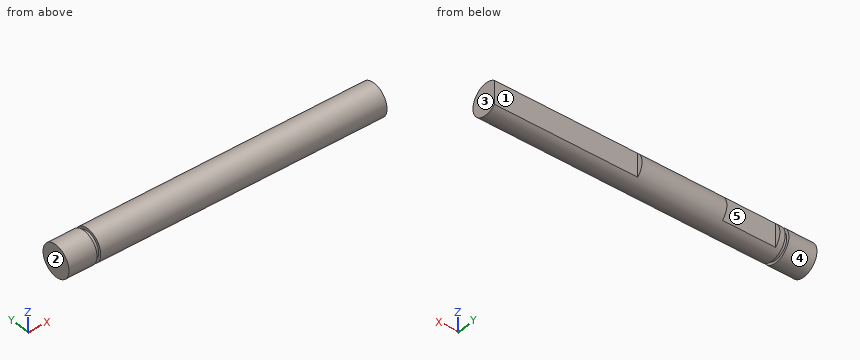
```python
from build123d import *

# Parameters (mm, degrees)
ESQUISSE2_W             = 10
ESQUISSE2_H             = 6
ESQUISSE2_W_2           = 27
ENL_V_MAT_EXTRU_1_DEPTH = 1


with BuildPart() as part:
    # Esquisse1 → Révolution1 (revolve)
    with BuildSketch(Plane.XY):
        Polygon((0, 0), (0, 3), (5.3, 3), (5.3, 2.5), (6, 2.5), (6, 3), (60, 3), (60, 0), align=None)
    revolve(axis=Axis((60, 0, 0), (-1, 0, 0)))

    # Esquisse2 → Enlèv. mat.-Extru.1 (cut)
    with BuildSketch(Plane(origin=(0, 3, 0), x_dir=(1, 0, 0), z_dir=(0, 1, 0))):
        with Locations((12, 0)):
            Rectangle(ESQUISSE2_W, ESQUISSE2_H)
        with Locations((46.5, 0)):
            Rectangle(ESQUISSE2_W_2, ESQUISSE2_H)
    extrude(amount=-ENL_V_MAT_EXTRU_1_DEPTH, mode=Mode.SUBTRACT)


solid = part.part
```
Could you check a few things on this model? Use its own coordinates, in mm. Face numbers are marked on the shaded views. A direction names the side the tool comes from. Coordinates: 2 decimals unless noted, no trailing zeros. Loops run counter-clockwise (first coordinate to the right, second up) from the corner with the lowest first, then second, coordinate; pieces in that order, holes last.
1) Thinking about a two-plate mould opening in X: for the marked faces 3, 4 and 5, which applies, released by +X, released by -X, zero draft, split by the parting line, or undercut?
Reported:
face 3: released by +X
face 4: zero draft
face 5: undercut
2) Imagine slicing it at D-D (y = -1.85). List the corners of the cut face in (x, z) for me, and give its area (3 significant figures).
Reported:
outline: (0, -2.36) - (5.3, -2.36) - (5.3, -1.68) - (6, -1.68) - (6, -2.36) - (60, -2.36) - (60, 2.36) - (6, 2.36) - (6, 1.68) - (5.3, 1.68) - (5.3, 2.36) - (0, 2.36) - close
area: 282 mm2
3) Will these pins go through, and if not, where does the flat tip stop? pin 1 Ø3.5 at (x, z) = (50.5, 0) entering from +Y; pin 2 Ø1.1 at (y, z) = (2.5, -1) entering from -X; pin 3 Ø0.5 at (y, z) = (2.5, 0.5) entering from +X.
Reported:
pin 1: stops at y = 2
pin 2: stops at x = 0
pin 3: stops at x = 33
4) Please list where these lines run through material, in increasing order: line 1 along X through (y, z) = (2.6, 1.15); line 2 along X through (y, z) = (-1.2, 2.4); line 3 along Y through (x, z) = (22, 0.15).
Reported:
line 1: x = 0 to 5.3, 6 to 7, 17 to 33
line 2: x = 0 to 5.3, 6 to 60
line 3: y = -3 to 3
5) Which directions (+Z, -Z, +X, -X, +Y, -Y) give clear straight access to the entire face, cutting with the end or side of a thin tool? Please do the marked faces 1 and 2.
Reported:
face 1: +Z, -Z, +X, +Y
face 2: +Z, -Z, -X, +Y, -Y
6) Imagine slicing it at B-B (y = 1.15). List the corners of the cut face in (x, z) for me.
Reported:
outline: (0, -2.77) - (5.3, -2.77) - (5.3, -2.22) - (6, -2.22) - (6, -2.77) - (60, -2.77) - (60, 2.77) - (6, 2.77) - (6, 2.22) - (5.3, 2.22) - (5.3, 2.77) - (0, 2.77) - close
7) Imagine slicing it at A-A (z = 0). List the corners of the cut face in (x, y) for me, and give its area (3 significant figures).
Reported:
outline: (0, -3) - (5.3, -3) - (5.3, -2.5) - (6, -2.5) - (6, -3) - (60, -3) - (60, 2) - (33, 2) - (33, 3) - (17, 3) - (17, 2) - (7, 2) - (7, 3) - (6, 3) - (6, 2.5) - (5.3, 2.5) - (5.3, 3) - (0, 3) - close
area: 322 mm2
8) Imagine slicing it at C-C (x = 23.5). List the corners of the cut face in (y, z) for me.
Reported:
outline: circle Ø6 at (0, 0)
